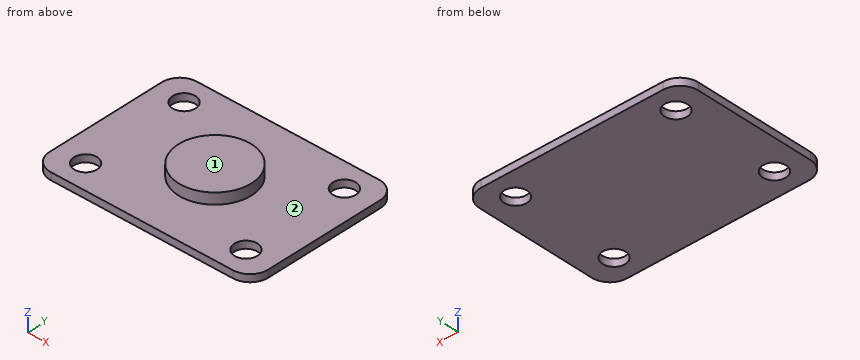
```python
from build123d import *

# Parameters (mm, degrees)
SKETCH_1_W          = 60
SKETCH_1_H          = 43
EXTRUDE_1_DEPTH     = 2
SKETCH_2_R          = 10
EXTRUDE_2_DEPTH     = 3
FILLET_1_R          = 5
SKETCH_3_R          = 3.15
CUT_EXTRUDE_1_DEPTH = 3


with BuildPart() as part:
    # 草图1 → 凸台-拉伸1 (new body)
    with BuildSketch(Plane.XY):
        Rectangle(SKETCH_1_W, SKETCH_1_H)
    extrude(amount=EXTRUDE_1_DEPTH)

    # 草图2 → 凸台-拉伸2 (add)
    with BuildSketch(Plane.XY.offset(2)):
        Circle(SKETCH_2_R)
    extrude(amount=EXTRUDE_2_DEPTH)

    # 圆角1
    fillet_1_edges = [part.edges().sort_by_distance(p)[0] for p in [
        (-30, 21.5, 1),
        (30, 21.5, 1),
        (30, -21.5, 1),
        (-30, -21.5, 1),
    ]]
    fillet(fillet_1_edges, radius=FILLET_1_R)

    # 草图3 → 切除-拉伸1 (cut)
    with BuildSketch(Plane(origin=(0, 0, 0), x_dir=(-1, 0, 0), z_dir=(0, 0, -1))):
        with Locations((22, 14.5)):
            Circle(SKETCH_3_R)
        with Locations((22, -14.5)):
            Circle(SKETCH_3_R)
        with Locations((-22, 14.5)):
            Circle(SKETCH_3_R)
        with Locations((-22, -14.5)):
            Circle(SKETCH_3_R)
    extrude(amount=-CUT_EXTRUDE_1_DEPTH, mode=Mode.SUBTRACT)


solid = part.part
```
Here's how the part is built. I have some questions about the finished solid (model axes, mm). Face numbers are marked on the shaded views. A direction names the side the tool comes from. Round coordinates to 2 decimals unless told otherwise and drop trailing zeros. Order: outer loops, then holes, each group sorted by start corner. A loop starts at its lowest first (then second) coordinate and runs counter-clockwise, first axis right, second up. Notation, with made-up numbers: M 12,88 L 51,88 A24 ccw 51,122 Z; hole C 28,81.5 d7. An arc over 180 degrees is marked long. Answer in a Markdown table with one row per item.
Item 1: Imagine slicing it at C-C, the plane z = 0.8. Write out the boundary of the cut face in (x, y).
A:
| item | result |
|---|---|
| outline | M -30,-16.5 A5 ccw -25,-21.5 L 25,-21.5 A5 ccw 30,-16.5 L 30,16.5 A5 ccw 25,21.5 L -25,21.5 A5 ccw -30,16.5 Z; hole C -22,-14.5 d6.3; hole C -22,14.5 d6.3; hole C 22,-14.5 d6.3; hole C 22,14.5 d6.3 |
Item 2: Imagine slicing it at A-A, the plane y = 14.5. Write out the boundary of the cut face in (x, z), and give its area (3 significant figures).
A:
| item | result |
|---|---|
| outline | M -30,0 L -25.15,0 L -25.15,2 L -30,2 Z; M -18.85,0 L 18.85,0 L 18.85,2 L -18.85,2 Z; M 25.15,0 L 30,0 L 30,2 L 25.15,2 Z |
| area | 94.8 mm2 |
Item 3: Imagine slicing it at B-B, the plane x = 22. Write out the boundary of the cut face in (y, z).
A:
| item | result |
|---|---|
| outline | M -21.5,0 L -17.65,0 L -17.65,2 L -21.5,2 Z; M -11.35,0 L 11.35,0 L 11.35,2 L -11.35,2 Z; M 17.65,0 L 21.5,0 L 21.5,2 L 17.65,2 Z |
Item 4: Imagine slicing it at D-D, the plane x = 0. Write out the boundary of the cut face in (y, z).
A:
| item | result |
|---|---|
| outline | M -21.5,0 L 21.5,0 L 21.5,2 L 10,2 L 10,5 L -10,5 L -10,2 L -21.5,2 Z |
Item 5: If I drill on L1, parallel to Y at x = -22, z = 0.75; L2, parallel to Y at x = 24, z = 0.7; L3, parallel to X at y = -14, z = 0.8, over which ranges is the centre line in solid material (lowest first)? Write a range as from..to.
A:
| item | result |
|---|---|
| L1 | y = -21.5..-17.65, -11.35..11.35, 17.65..21.5 |
| L2 | y = -21.5..-16.93, -12.07..12.07, 16.93..21.5 |
| L3 | x = -30..-25.11, -18.89..18.89, 25.11..30 |
Item 6: For the marked faces 1 and 2, which set-ups out of +Z, -Z, +X, -X, +Y, -Y let a thin tool reach every point of the face, with its end or its side?
A:
| item | result |
|---|---|
| face 1 | +Z, +X, -X, +Y, -Y |
| face 2 | +Z |
Item 7: I'm going to push a flat-ended pin straight in: pin 1 (1.5 mm diameter, centred on x = -21.5, y = -4.5, fed in from +Z). Where does the tip first touch, or does it pass through?
A:
| item | result |
|---|---|
| pin 1 | stops at z = 2 |
